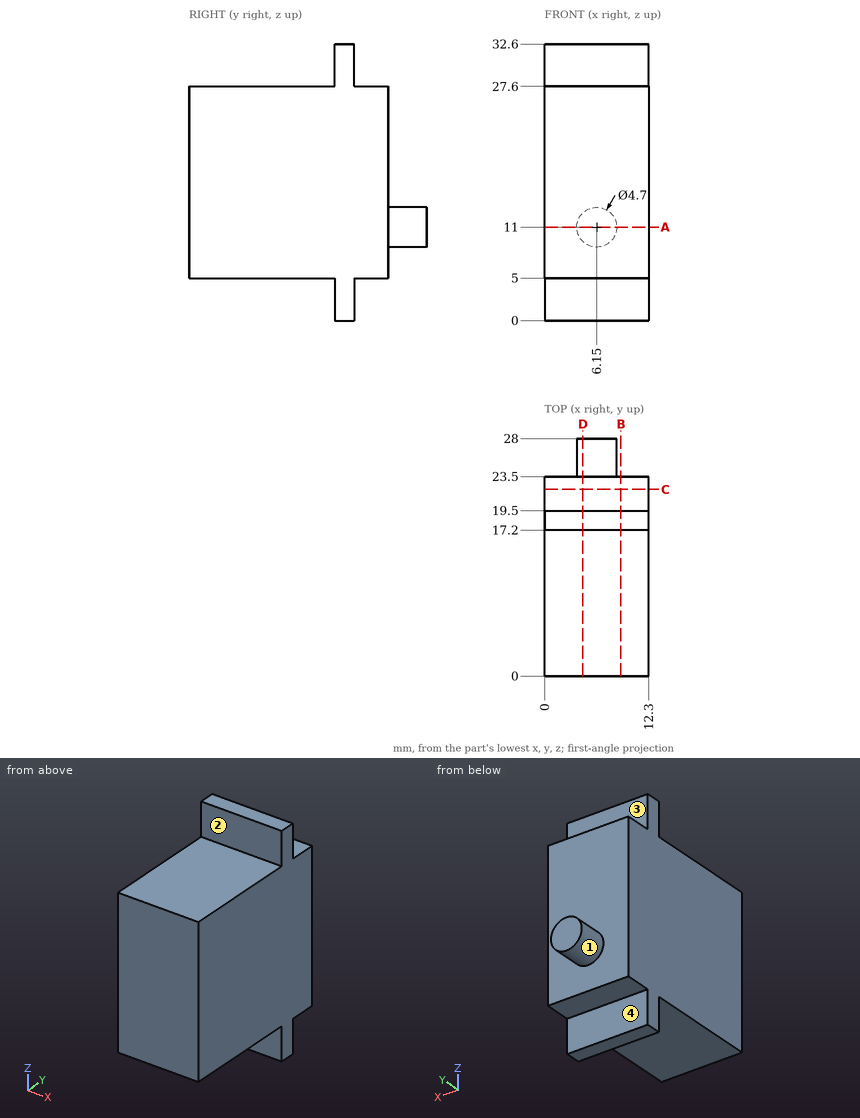
Part print with two shaded views. Sizes in mm from the minimum x, y, z corner. A direction names the side the tool comes from. Give positions to 0.01 mm unless a question says otherwise; leave off trailing zeros. Order: outer loops, then holes, each group sorted by start corner. A loop starts at its lowest first (then second) coordinate and runs counter-clockwise, first axis right, second up. Notation, with made-up numbers: (62.5, 80.25) - (107.5, 80.25) arc R27 cw to (107.5, 110.25) - close; hole circle Ø6 at (-36, 27). An arc over 180 degrees is marked (long way). Write each question's results on one line, items separated by ' | '.
1. Pin check, flat tips, straight feed: pin 1 (4 mm diameter, centred on x = 8.5, z = 2, fed in from +Y); pin 2 (3.5 mm diameter, centred on x = 3.5, y = 9.5, fed in from -Z); pin 3 (1.5 mm diameter, centred on x = 5.5, z = 31, fed in from -Y). Stop position of each tip, or through.
Calculated:
pin 1: stops at y = 19.5 | pin 2: stops at z = 5 | pin 3: stops at y = 17.2
2. Saw through at B-B on x = 9. List the corners of the cut face in (y, z), and give its area (3 significant figures).
Calculated:
outline: (0, 5) - (17.2, 5) - (17.2, 0) - (19.5, 0) - (19.5, 5) - (23.5, 5) - (23.5, 27.6) - (19.5, 27.6) - (19.5, 32.6) - (17.2, 32.6) - (17.2, 27.6) - (0, 27.6) - close | area: 554 mm2
3. Saw through at D-D on x = 4.5. List the corners of the cut face in (y, z), and give its area (3 significant figures).
Calculated:
outline: (0, 5) - (17.2, 5) - (17.2, 0) - (19.5, 0) - (19.5, 5) - (23.5, 5) - (23.5, 9.33) - (28, 9.33) - (28, 12.67) - (23.5, 12.67) - (23.5, 27.6) - (19.5, 27.6) - (19.5, 32.6) - (17.2, 32.6) - (17.2, 27.6) - (0, 27.6) - close | area: 569 mm2
4. Probe L1, parallel to Y at x = 7.25, z = 7.5; L2, parallel to Z at x = 10, y = 8.25; L3, parallel to Y at x = 10, z = 28. List the from-to ranges inside material, lowest first. Write a range as from..to.
Calculated:
L1: y = 0..23.5 | L2: z = 5..27.6 | L3: y = 17.2..19.5
5. Saw through at C-C on y = 22. List the corners of the cut face in (x, z).
Calculated:
outline: (0, 5) - (12.3, 5) - (12.3, 27.6) - (0, 27.6) - close
6. 3-axis set-ups, long thin cutter, end or side, ignore diameter. For the marked faces 1, 2, 3 and 4: which of +Z, -Z, +X, -X, +Y, -Y reach the whole face in a straight line?
Calculated:
face 1: +Y | face 2: +Z, +X, -X, -Y | face 3: +Z, +X, -X, +Y | face 4: -Z, +X, -X, +Y
7. Saw through at A-A on z = 11. List the corners of the cut face in (x, y).
Calculated:
outline: (0, 0) - (12.3, 0) - (12.3, 23.5) - (8.5, 23.5) - (8.5, 28) - (3.8, 28) - (3.8, 23.5) - (0, 23.5) - close
